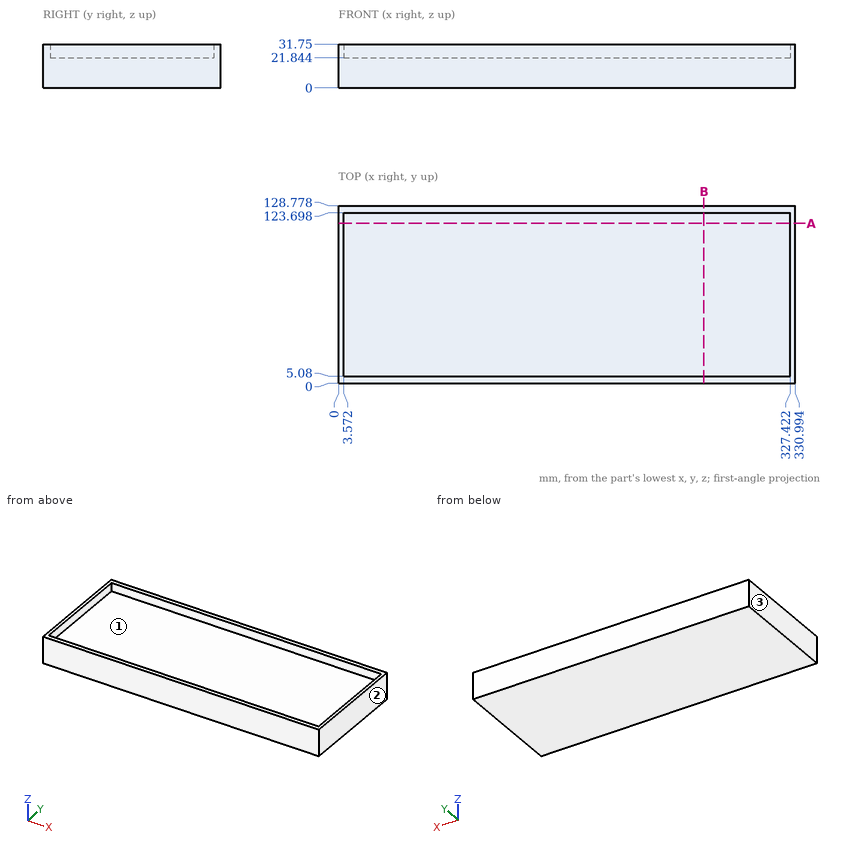
Check sheet for the drawn part. Datum: minimum x, y, z corner. Units: mm. Round coordinates to 2 decimals unless told otherwise and drop trailing zeros. Order: outer loops, then holes, each group sorted by start corner. A loop starts at its lowest first (then second) coordinate and runs counter-clockwise, first axis right, second up.
1) Section check B-B (x = 265). Record the boundary of the cut face in (y, z), and give its area (3 significant figures).
2) Scan lines: line 1 (Y direction, x = 47, z = 23); line 2 (X direction, y = 60, z = 28); line 3 (Z direction, x = 229, y = 26.5). Record each from-to range of solid material in increasing order.
3) Section check A-A (y = 116). Record the boundary of the cut face in (x, z), and give its area (3 significant figures).
4) Go/stop test with flat-tipped pins: pin 1 Ø8 at (x, y) = (210, 22.5) entering from +Z; pin 2 Ø2 at (x, y) = (244, 69) entering from -Z. Record where each tip stops, or that it passes through.
5) Mould release check, pull along X, two halves, no side actions. Record for the marked faces 1, 2 and 3: +X half, -X half, draft (parallel to the pull), parting line (faces both ways), or undercut.
Result:
1. outline: (0, 0) - (128.78, 0) - (128.78, 31.75) - (123.7, 31.75) - (123.7, 21.84) - (5.08, 21.84) - (5.08, 31.75) - (0, 31.75) - close
1. area: 2,910 mm2
2. line 1: y = 0 to 5.08, 123.7 to 128.78
2. line 2: x = 0 to 3.57, 327.42 to 330.99
2. line 3: z = 0 to 21.84
3. outline: (0, 0) - (330.99, 0) - (330.99, 31.75) - (327.42, 31.75) - (327.42, 21.84) - (3.57, 21.84) - (3.57, 31.75) - (0, 31.75) - close
3. area: 7,300 mm2
4. pin 1: stops at z = 21.84
4. pin 2: stops at z = 0
5. face 1: undercut
5. face 2: +X half
5. face 3: -X half
